```python
from build123d import *

# Parameters (mm, degrees)
SKETCH1_R             = 4.5
SKETCH1_R_2           = 1.05
BOSS_EXTRUDE1_DEPTH   = 8
BOSS_EXTRUDE1_2_DEPTH = 8
BOSS_EXTRUDE1_3_DEPTH = 8
BOSS_EXTRUDE1_4_DEPTH = 8
BOSS_EXTRUDE2_REACH   = 91.358
SKETCH2_W             = 3
SKETCH2_H             = 27.5
CUT_EXTRUDE1_DEPTH    = 54.46973443
SKETCH4_W             = 59.9
SKETCH4_H             = 22.9
SKETCH4_W_2           = 51.9
SKETCH4_H_2           = 14.9
BOSS_EXTRUDE3_DEPTH   = 2
SKETCH7_W             = 9.5
SKETCH7_H             = 3
BOSS_EXTRUDE5_DEPTH   = 4.3
CUT_EXTRUDE3_START    = -1
SKETCH8_W             = 5.5
SKETCH8_H             = 5.5
CUT_EXTRUDE3_DEPTH    = 1.8
CHAMFER3_SIZE         = 3
SKETCH9_R             = 1.55
CUT_EXTRUDE4_DEPTH    = 5.4
BOSS_EXTRUDE6_DEPTH   = 4
SKETCH11_R            = 1.5
BOSS_EXTRUDE7_DEPTH   = 0.5
FILLET2_R             = 3
CHAMFER4_SIZE         = 1
CHAMFER5_SIZE         = 2
SKETCH12_W            = 5.5
SKETCH12_H            = 1.8
CUT_EXTRUDE5_DEPTH    = 0.1


with BuildPart() as part:
    # Sketch1 → Boss-Extrude1 (new body)
    with BuildSketch(Plane(origin=(0, 0, 0), x_dir=(1, 0, 0), z_dir=(0, 1, 0))):
        with Locations(Location((27.95, -56.4, 0), (0, 0, 270))):
            Circle(SKETCH1_R)
        with Locations(Location((27.95, -56.4, 0), (0, 0, 270))):
            Circle(SKETCH1_R_2, mode=Mode.SUBTRACT)
    extrude(amount=BOSS_EXTRUDE1_DEPTH)



with BuildPart() as body_2:
    # Sketch1 → Boss-Extrude1 2 (new body)
    with BuildSketch(Plane(origin=(0, 0, 0), x_dir=(1, 0, 0), z_dir=(0, 1, 0))):
        with Locations(Location((-27.95, -56.4, 0), (0, 0, 270))):
            Circle(SKETCH1_R)
        with Locations(Location((-27.95, -56.4, 0), (0, 0, 270))):
            Circle(SKETCH1_R_2, mode=Mode.SUBTRACT)
    extrude(amount=BOSS_EXTRUDE1_2_DEPTH)


with BuildPart() as body_3:
    # Sketch1 → Boss-Extrude1 3 (new body)
    with BuildSketch(Plane(origin=(0, 0, 0), x_dir=(1, 0, 0), z_dir=(0, 1, 0))):
        with BuildLine():
            Line((-32.45, -37.5), (-32.45, -25.5))
            Line((-32.45, -25.5), (-23.45, -25.5))
            Line((-23.45, -25.5), (-23.45, -37.5))
            ThreePointArc((-23.45, -37.5), (-27.95, -42), (-32.45, -37.5))
        make_face()
        with Locations(Location((-27.95, -37.5, 0), (0, 0, 270))):
            Circle(SKETCH1_R_2, mode=Mode.SUBTRACT)
    extrude(amount=BOSS_EXTRUDE1_3_DEPTH)

    # Boss-Extrude2: up to this face of the body (flat: up to its plane)
    boss_extrude2_end = Plane(body_3.part.faces().sort_by_distance((-32.45, 4, 31.5))[0])
    # Sketch2 → Boss-Extrude2 (add, up to the picked face)
    with BuildSketch(Plane(origin=(32.45, 0, 0), x_dir=(0, 0, -1), z_dir=(1, 0, 0)), mode=Mode.PRIVATE) as boss_extrude2_sk1:
        with Locations((-27, 13.75)):
            Rectangle(SKETCH2_W, SKETCH2_H)
    boss_extrude2_tool1 = split(extrude(boss_extrude2_sk1.sketch, amount=-BOSS_EXTRUDE2_REACH, mode=Mode.PRIVATE), bisect_by=boss_extrude2_end, keep=Keep.BOTH, mode=Mode.PRIVATE)


with BuildPart() as body_4:
    # Sketch1 → Boss-Extrude1 4 (new body)
    with BuildSketch(Plane(origin=(0, 0, 0), x_dir=(1, 0, 0), z_dir=(0, 1, 0))):
        with BuildLine():
            Line((32.45, -37.5), (32.45, -25.5))
            Line((32.45, -25.5), (23.45, -25.5))
            Line((23.45, -25.5), (23.45, -37.5))
            ThreePointArc((23.45, -37.5), (27.95, -42), (32.45, -37.5))
        make_face()
        with Locations(Location((27.95, -37.5, 0), (0, 0, 270))):
            Circle(SKETCH1_R_2, mode=Mode.SUBTRACT)
    extrude(amount=BOSS_EXTRUDE1_4_DEPTH)


with BuildPart() as body_3_1:
    add(body_3.part)

    add(body_4.part)  # Boss-Extrude2 merges body 4
    add(boss_extrude2_tool1.solids().sort_by(Axis((32.45, 13.75, 27), (-1, 0, 0)))[0])

    # Sketch3 → Cut-Extrude1 (cut, through all)
    with BuildSketch(Plane.XY.offset(28.5)):
        Polygon((-32.45, 8), (-9, 27.5), (-32.45, 27.5), align=None)
        Polygon((9, 27.5), (32.45, 8), (32.45, 27.5), align=None)
        Polygon((-23.45, 8), (-23.45, 0), (23.45, 0), (23.45, 8), (9.620512821, 19.5), (-9.620512821, 19.5), align=None)
    extrude(amount=-CUT_EXTRUDE1_DEPTH, mode=Mode.SUBTRACT)


with BuildPart() as part_1:
    add(part.part)

    add(body_2.part)  # Boss-Extrude3 merges body 2

    add(body_3_1.part)  # Boss-Extrude3 merges body 3
    # Sketch4 → Boss-Extrude3 (add)
    with BuildSketch(Plane.XZ):
        with Locations((0, 46.95)):
            Rectangle(SKETCH4_W, SKETCH4_H)
        with Locations((0, 46.95)):
            Rectangle(SKETCH4_W_2, SKETCH4_H_2, mode=Mode.SUBTRACT)
    extrude(amount=-BOSS_EXTRUDE3_DEPTH)

    # Sketch7 → Boss-Extrude5 (add)
    with BuildSketch(Plane(origin=(0, 27.5, 0), x_dir=(1, 0, 0), z_dir=(0, 1, 0))):
        with Locations((0, -30)):
            Rectangle(SKETCH7_W, SKETCH7_H)
    extrude(amount=-BOSS_EXTRUDE5_DEPTH)

    # Sketch8 → Cut-Extrude3 (cut)
    with BuildSketch(Plane(origin=(0, 27.5, 0), x_dir=(1, 0, 0), z_dir=(0, 1, 0)).offset(CUT_EXTRUDE3_START)):
        with Locations((0, -28.75)):
            Rectangle(SKETCH8_W, SKETCH8_H)
    extrude(amount=-CUT_EXTRUDE3_DEPTH, mode=Mode.SUBTRACT)

    # Chamfer3
    chamfer3_edges = [part_1.edges().sort_by_distance(p)[0] for p in [
        (0, 23.2, 28.5),
    ]]
    chamfer(chamfer3_edges, length=CHAMFER3_SIZE - 0.0001)  # a hair under: the kernel refuses the full size

    # Sketch9 → Cut-Extrude4 (cut)
    with BuildSketch(Plane(origin=(0, 27.5, 0), x_dir=(1, 0, 0), z_dir=(0, 1, 0))):
        with Locations(Location((0, -28.75, 0), (0, 0, 270))):
            Circle(SKETCH9_R)
    extrude(amount=-CUT_EXTRUDE4_DEPTH, mode=Mode.SUBTRACT)

    # Sketch10 → Boss-Extrude6 (add)
    with BuildSketch(Plane.XZ):
        with BuildLine():
            Line((-32.45, 25.5), (-35.2, 25.5))
            ThreePointArc((-35.2, 25.5), (-40.990483074, 29.928279361), (-38.233673919, 36.676564744))
            Line((-38.233673919, 36.676564744), (-29.95, 41.531128874))
            Line((-29.95, 41.531128874), (-29.95, 25.5))
            Line((-29.95, 25.5), (-32.45, 25.5))
        make_face()
        Polygon((-35.2, 28.324573519), (-32.45, 29.91228676), (-32.45, 33.08771324), (-35.2, 34.675426481), (-37.95, 33.08771324), (-37.95, 29.91228676), align=None, mode=Mode.SUBTRACT)
    boss_extrude6 = extrude(amount=-BOSS_EXTRUDE6_DEPTH)

    # Sketch11 → Boss-Extrude7 (add)
    with BuildSketch(Plane.XZ):
        Polygon((-37.95, 33.08771324), (-37.95, 29.91228676), (-35.2, 28.324573519), (-32.45, 29.91228676), (-32.45, 33.08771324), (-35.2, 34.675426481), align=None)
        with Locations(Location((-35.2, 31.5, 0), (0, 0, 270))):
            Circle(SKETCH11_R, mode=Mode.SUBTRACT)
    boss_extrude7 = extrude(amount=-BOSS_EXTRUDE7_DEPTH)

    # Mirror1: Boss-Extrude6, Boss-Extrude7 across plane
    add(boss_extrude6.mirror(Plane(origin=(0, 0, 0), x_dir=(0, 0, 1), z_dir=(1, 0, 0))))
    add(boss_extrude7.mirror(Plane(origin=(0, 0, 0), x_dir=(0, 0, 1), z_dir=(1, 0, 0))))

    # Fillet2
    fillet2_edges = [part_1.edges().sort_by_distance(p)[0] for p in [
        (23.918871126, 1, 58.4),
        (-25.95, 1, 52.368871126),
        (-23.918871126, 1, 58.4),
        (-29.95, 1, 52.368871126),
        (-23.918871126, 1, 54.4),
        (23.918871126, 1, 39.5),
        (-23.918871126, 1, 39.5),
        (23.45, 1, 35.5),
        (-23.45, 1, 35.5),
        (25.95, 1, 52.368871126),
        (-25.95, 1, 41.531128874),
        (29.95, 1, 52.368871126),
        (25.95, 1, 41.531128874),
        (23.918871126, 1, 54.4),
    ]]
    fillet(fillet2_edges, radius=FILLET2_R)

    # Chamfer4
    chamfer4_edges = [part_1.edges().sort_by_distance(p)[0] for p in [
        (23.45, 4, 25.5),
        (-23.45, 4, 25.5),
    ]]
    chamfer(chamfer4_edges, length=CHAMFER4_SIZE)

    # Chamfer5
    chamfer5_edges = [part_1.edges().sort_by_distance(p)[0] for p in [
        (27.95, 8, 51.9),
        (-27.95, 8, 51.9),
        (-32.45, 8, 33),
        (-27.95, 8, 42),
        (-23.45, 8, 33),
        (23.45, 8, 33),
        (27.95, 8, 42),
        (32.45, 8, 33),
    ]]
    chamfer(chamfer5_edges, length=CHAMFER5_SIZE)

    # Sketch12 → Cut-Extrude5 (cut)
    with BuildSketch(Plane.XY.offset(26)):
        with Locations((0, 25.6)):
            Rectangle(SKETCH12_W, SKETCH12_H)
    extrude(amount=-CUT_EXTRUDE5_DEPTH, mode=Mode.SUBTRACT)


solid = part_1.part
```
The listing builds one solid part. Answer for the finished solid, in the listing's coordinates (mm). A direction names the side the tool comes from. Round coordinates to 2 decimals unless told otherwise and drop trailing zeros. Order: outer loops, then holes, each group sorted by start corner. A loop starts at its lowest first (then second) coordinate and runs counter-clockwise, first axis right, second up. Notation, with made-up numbers: (18, 65.25) -> (60, 65.25) arc R19 ccw to (60, 92.25) -> close; hole circle Ø8 at (-0.75, 10.25). An arc over 180 degrees is marked (long way). Answer as CSV lines item,"result".
Q1. A cutting plane is placed at D-D on x = -19. Determine the outline of the cut face in (y, z), plus the area to 3 significant figures.
Computed values:
outline,"(0, 35.5) -> (2, 35.5) -> (2, 39.5) -> (0, 39.5) -> close; (0, 54.4) -> (2, 54.4) -> (2, 58.4) -> (0, 58.4) -> close; (11.7, 25.5) -> (19.18, 25.5) -> (19.18, 28.5) -> (11.7, 28.5) -> close"
area,"38.5 mm^2"
Q2. Given pin 1 (1.6 mm diameter, centred on y = 1.5, z = 31, fed in from +X); pin 2 (2.5 mm diameter, centred on x = -27.95, z = 37.5, fed in from +Y); pin 3 (10 mm diameter, centred on y = 22.5, z = 30.5, fed in from +X); pin 4 (2 mm diameter, centred on y = 5.5, z = 31.5, fed in from +X), each flat-ended and moving along its own axis, determine where each tip first touches the part or whether it passes through.
Computed values:
pin 1,"stops at x = 41.2"
pin 2,"stops at y = 8"
pin 3,"stops at x = 20.52"
pin 4,"stops at x = 32.45"
Q3. A cutting plane is placed at C-C on y = 14.75. Determine the outline of the cut face in (x, z).
Computed values:
outline,"(-24.33, 25.5) -> (-15.33, 25.5) -> (-15.33, 28.5) -> (-24.33, 28.5) -> close; (15.33, 25.5) -> (24.33, 25.5) -> (24.33, 28.5) -> (15.33, 28.5) -> close"
Q4. Which of the six approach directions +Z, -Z, +X, -X, +Y, -Y give full straight-line access (tool end or side, diameter ignored) to faces 1 (the flat face through (4.75, 25, 30)), 2 (the flat face through (-29.95, 1, 46)), 3 (the flat face through (0, 1, 58.4)), 4 (the cylindrical face through (-0.594, 27.007, 30.182))?
Computed values:
face 1,"+Z, +X, +Y, -Y"
face 2,"-X, +Y, -Y"
face 3,"+Z, +Y, -Y"
face 4,"+Y"
Q5. For a pull along X with two mould halves and no side action, classify faces 5 (the cylindrical face through (22.55, 1.01, 34.64)), 6 (the flat face through (27.4, 8, 57.5)), 7 (the flat face through (20.561, 17.886, 27.021)) as +X half, -X half, draft (parallel to the pull), parting line (faces both ways), or undercut.
Computed values:
face 5,"undercut"
face 6,"draft"
face 7,"+X half"
Q6. Consider line 1 (Z direction, x = 27.95, y = 4.55); line 2 (X direction, y = 5.95, z = 37.5); line 3 (X direction, y = 0.15, z = 31.5). Determine where each line is inside the solid, lowest interval first. Write a range as from..to.
Computed values:
line 1,"z = 25.5..36.45, 38.55..42, 51.9..55.35, 57.45..60.9"
line 2,"x = -32.45..-29, -26.9..-23.45, 23.45..26.9, 29..32.45"
line 3,"x = -41.2..-36.7, -33.7..-23.45, 23.45..33.7, 36.7..41.2"
Q7. A cutting plane is placed at B-B on z = 56.4. Determine the outline of the cut face in (x, y), plus the area to 3 significant figures.
Computed values:
outline,"(-32.45, 0) -> (32.45, 0) -> (32.45, 6) -> (30.45, 8) -> (29, 8) -> (29, 2) -> (26.9, 2) -> (26.9, 8) -> (25.45, 8) -> (23.45, 6) -> (23.45, 2) -> (-23.45, 2) -> (-23.45, 6) -> (-25.45, 8) -> (-26.9, 8) -> (-26.9, 2) -> (-29, 2) -> (-29, 8) -> (-30.45, 8) -> (-32.45, 6) -> close"
area,"205 mm^2"
Q8. A cutting plane is placed at A-A on x = -7.5. Determine the outline of the cut face in (y, z).
Computed values:
outline,"(0, 35.5) -> (2, 35.5) -> (2, 39.5) -> (0, 39.5) -> close; (0, 54.4) -> (2, 54.4) -> (2, 58.4) -> (0, 58.4) -> close; (19.5, 25.5) -> (27.5, 25.5) -> (27.5, 28.5) -> (19.5, 28.5) -> close"
